Input: part model. Units: mm. Frame: model coordinates. Face numbers are marked on the shaded views. A direction names the side the tool comes from. Give positions to 0.01 mm unless a question says otherwise; leave off trailing zeros. Loops run counter-clockwise (first coordinate to the right, second up) from the corner with the lowest first, then second, coordinate; pieces in that order, holes last. Notation, with made-up numbers: (-24, 85) - (-11, 85) arc R23 ccw to (-11, 110) - close; hole circle Ø9 at (63, -3). An arc over 180 degrees is marked (long way). One line per item, written item: value.
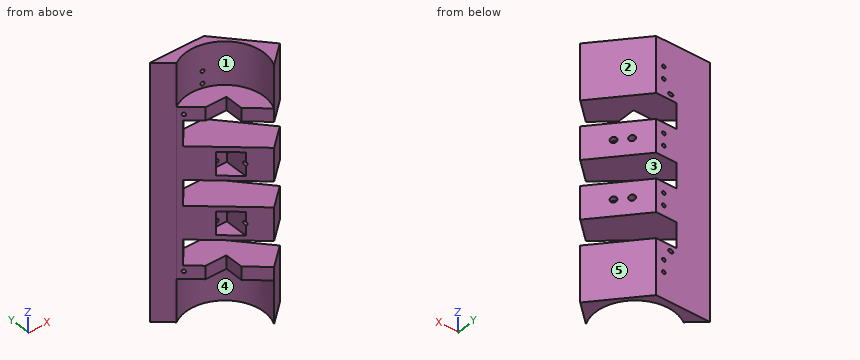
from build123d import *

# Parameters (mm, degrees)
EXTRUDE_1_DEPTH      = 250
SKETCH_2_R           = 38.7
CUT_EXTRUDE_1_DEPTH  = 42
SKETCH_3_W           = 28.23457759
SKETCH_3_H           = 26.953334418
CUT_EXTRUDE_2_DEPTH  = 14
SKETCH_4_W           = 170
SKETCH_4_H           = 25
CUT_EXTRUDE_3_DEPTH  = 78
SKETCH_7_R           = 1.75
CUT_EXTRUDE_5_DEPTH  = 25
SKETCH_6_R           = 1.75
CUT_EXTRUDE_6_DEPTH  = 90
SKETCH_5_R           = 1.75
CUT_EXTRUDE_8_DEPTH  = 10
SKETCH_9_R           = 1.75
CUT_EXTRUDE_9_DEPTH  = 124
SKETCH_10_W          = 17.333433977
SKETCH_10_H          = 22.880132851
CUT_EXTRUDE_10_DEPTH = 31
SKETCH_11_R          = 3
CUT_EXTRUDE_11_DEPTH = 10


with BuildPart() as part:
    # 草图1 → 凸台-拉伸1 (new body)
    with BuildSketch(Plane.XY):
        Polygon((0, 0), (53, 0), (92.057126275, -44.146050576), (71.602312757, -62.242940876), (15.094191604, -13.12118058), align=None)
    extrude(amount=EXTRUDE_1_DEPTH)

    # 草图2 → 切除-拉伸1 (cut)
    with BuildSketch(Plane.XY.offset(250)):
        with Locations((36.7, -45.33)):
            Circle(SKETCH_2_R)
    cut_extrude_1 = extrude(amount=-CUT_EXTRUDE_1_DEPTH, mode=Mode.SUBTRACT)

    # 草图3 → 切除-拉伸2 (cut)
    with BuildSketch(Plane.XY.offset(208)):
        with Locations((38.582711205, -41.306667209)):
            Rectangle(SKETCH_3_W, SKETCH_3_H)
    cut_extrude_2 = extrude(amount=-CUT_EXTRUDE_2_DEPTH, mode=Mode.SUBTRACT)

    # 草图4 → 切除-拉伸3 (cut)
    with BuildSketch(Plane(origin=(0, 0, 0), x_dir=(0.75470958, -0.656059029, 0), z_dir=(-0.656059029, -0.75470958, 0))):
        with Locations((110, 67.5)):
            Rectangle(SKETCH_4_W, SKETCH_4_H)
        with Locations((110, 125)):
            Rectangle(SKETCH_4_W, SKETCH_4_H)
        with Locations((110, 182.5)):
            Rectangle(SKETCH_4_W, SKETCH_4_H)
    extrude(amount=-CUT_EXTRUDE_3_DEPTH, mode=Mode.SUBTRACT)

    # 镜向1: 切除-拉伸1, 切除-拉伸2 across plane
    add(cut_extrude_1.mirror(Plane.XY.offset(125)), mode=Mode.SUBTRACT)
    add(cut_extrude_2.mirror(Plane.XY.offset(125)), mode=Mode.SUBTRACT)

    # 草图7 → 切除-拉伸5 (cut)
    with BuildSketch(Plane(origin=(0, 0, 0), x_dir=(1, 0, 0), z_dir=(0, 1, 0))):
        with Locations((45.5, -159.75)):
            Circle(SKETCH_7_R)
        with Locations((45.5, -147.75)):
            Circle(SKETCH_7_R)
        with Locations((45.5, -102.25)):
            Circle(SKETCH_7_R)
        with Locations((45.5, -90.25)):
            Circle(SKETCH_7_R)
    extrude(amount=-CUT_EXTRUDE_5_DEPTH, mode=Mode.SUBTRACT)

    # 草图6 → 切除-拉伸6 (cut)
    with BuildSketch(Plane(origin=(0, 0, 0), x_dir=(0.75470958, -0.656059029, 0), z_dir=(-0.656059029, -0.75470958, 0))):
        with Locations((72.838810202, 96.25)):
            Circle(SKETCH_6_R)
        with Locations((58.538810202, 96.25)):
            Circle(SKETCH_6_R)
        with Locations((72.838810202, 153.75)):
            Circle(SKETCH_6_R)
        with Locations((58.538810202, 153.75)):
            Circle(SKETCH_6_R)
    extrude(amount=-CUT_EXTRUDE_6_DEPTH, mode=Mode.SUBTRACT)

    # 草图5 → 切除-拉伸8 (cut)
    with BuildSketch(Plane(origin=(0, 0, 0), x_dir=(1, 0, 0), z_dir=(0, 1, 0))):
        with Locations((45.5, -212.3)):
            Circle(SKETCH_5_R)
        with Locations((45.5, -224.3)):
            Circle(SKETCH_5_R)
        with Locations((45.5, -25.7)):
            Circle(SKETCH_5_R)
        with Locations((45.5, -37.7)):
            Circle(SKETCH_5_R)
    extrude(amount=-CUT_EXTRUDE_8_DEPTH, mode=Mode.SUBTRACT)

    # 草图9 → 切除-拉伸9 (cut)
    with BuildSketch(Plane(origin=(29.7295376, 26.302473018, 0), x_dir=(0, 0, -1), z_dir=(0.748955721, 0.662620048, 0))):
        with Locations((-49.264197296, -25.601913803)):
            Circle(SKETCH_9_R)
        with Locations((-200.735802704, -25.601913803)):
            Circle(SKETCH_9_R)
    extrude(amount=-CUT_EXTRUDE_9_DEPTH, mode=Mode.SUBTRACT)

    # 草图10 → 切除-拉伸10 (cut)
    with BuildSketch(Plane(origin=(0, -25, 0), x_dir=(1, 0, 0), z_dir=(0, 1, 0))):
        with Locations((46.622123833, -96.2830381)):
            Rectangle(SKETCH_10_W, SKETCH_10_H)
    cut_extrude_10 = extrude(amount=-CUT_EXTRUDE_10_DEPTH, mode=Mode.SUBTRACT)

    # 镜向2: 切除-拉伸10 across plane
    add(cut_extrude_10.mirror(Plane.XY.offset(125)), mode=Mode.SUBTRACT)

    # 草图11 → 切除-拉伸11 (cut)
    with BuildSketch(Plane(origin=(22.962066015, 26.414835308, 0), x_dir=(-0.75470958, 0.656059029, 0), z_dir=(-0.656059029, -0.75470958, 0))):
        with Locations((-58.538810202, -96.25)):
            Circle(SKETCH_11_R)
        with Locations((-72.838810202, -96.25)):
            Circle(SKETCH_11_R)
        with Locations((-58.538810202, -153.75)):
            Circle(SKETCH_11_R)
        with Locations((-72.838810202, -153.75)):
            Circle(SKETCH_11_R)
    extrude(amount=CUT_EXTRUDE_11_DEPTH, mode=Mode.SUBTRACT)


solid = part.part
Item 1: Pin query (flat end, axial travel): P1, Ø14, axis at x = 46, z = 95, coming from the -Y side; P2, Ø5, axis at x = 48.5, y = -36.5, coming from the -Z side; P3, Ø18.5, axis at y = -40, z = 157, coming from the -X side. Return the tip coordinate at first contact, or that it passes through.
Verdict:
P1: stops at y = -25
P2: stops at z = 80
P3: stops at x = 35.37
Item 2: Access query for the marked faces 4 and 5. Directions: +Z, -Z, +X, -X, +Y, -Y. A direction counts if a zero-diameter tool reaches every point of the face in a straight line with its end or side. Return the directions, or none.
Verdict:
face 4: -Z
face 5: +Z, -Z, +X, +Y
Item 3: Material intervals for L1, parallel to Z at x = 48, y = -11.5; L2, parallel to Z at x = 65, y = -14; L3, parallel to X at y = -13, z = 159, sorted ascending.
Verdict:
L1: z = 42 to 55, 80 to 112.5, 137.5 to 170, 195 to 208
L2: z = 0 to 55, 80 to 93.26, 99.24 to 112.5, 137.5 to 150.76, 156.74 to 170, 195 to 250
L3: x = 14.95 to 43.92, 47.08 to 64.5
Item 4: Section B-B, the plane z = 33. Output: boundary loops of the cut face in (x, y).
Verdict:
outline: (0, 0) - (15.16, -13.18) arc R38.7 cw to (71.54, -62.19) - (71.6, -62.24) - (92.06, -44.15) - (53, 0) - close
Item 5: Section C-C, the plane y = -4. Count the separate pieces of the cut face and the enclosed holes in it, and give its area (3 significant figures).
Verdict:
separate pieces: 1
enclosed holes: 10
area: 10,900 mm^2
Item 6: Draft query along Y for the marked faces 1, 2 and 3. Return one class per face: pulls with the +Y half, pulls with the -Y half, needs draft (parallel to the pull), parting line crosses it, or undercut.
Verdict:
face 1: undercut
face 2: pulls with the +Y half
face 3: needs draft
Item 7: Section A-A, the plane y = -51.5. Output: boundary loops of the cut face in (x, z) (3 decimals).
Verdict:
outline: (59.244, 42) - (74.905, 42) - (74.905, 0) - (83.745, 0) - (83.745, 55) - (59.244, 55) - close; (59.244, 80) - (83.745, 80) - (83.745, 112.5) - (59.244, 112.5) - close; (59.244, 137.5) - (83.745, 137.5) - (83.745, 170) - (59.244, 170) - close; (59.244, 195) - (83.745, 195) - (83.745, 250) - (74.905, 250) - (74.905, 208) - (59.244, 208) - close
